from build123d import *

# Parameters (mm, degrees)
F0_R     = 1.75
F1_DEPTH = 1.6
F2_W     = 5.842995
F2_H     = 15.024841
F3_DEPTH = 8
F4_W     = 32
F4_H     = 50
F5_DEPTH = 19
F6_W     = 3
F6_H     = 14
F7_DEPTH = 32
F8_W     = 8.602944
F8_H     = 27.794118
F9_DEPTH = 14


with BuildPart() as f1:
    # F0 (on Top) → F1 (new body)
    with BuildSketch(Plane.XY):
        with BuildLine():
            ThreePointArc((35.5, 25), (34.62132, 27.12132), (32.5, 28))
            Line((32.5, 28), (-32.5, 28))
            ThreePointArc((-32.5, 28), (-34.62132, 27.12132), (-35.5, 25))
            Line((-35.5, 25), (-35.5, -25))
            ThreePointArc((-35.5, -25), (-34.62132, -27.12132), (-32.5, -28))
            Line((-32.5, -28), (32.5, -28))
            ThreePointArc((32.5, -28), (34.62132, -27.12132), (35.5, -25))
            Line((35.5, -25), (35.5, 25))
        make_face()
        with Locations((-32.5, -25)):
            Circle(F0_R, mode=Mode.SUBTRACT)
        with Locations((32.5, -25)):
            Circle(F0_R, mode=Mode.SUBTRACT)
        with Locations((-32.5, 25)):
            Circle(F0_R, mode=Mode.SUBTRACT)
        with Locations((32.5, 25)):
            Circle(F0_R, mode=Mode.SUBTRACT)
    extrude(amount=F1_DEPTH)

    # F2 (on face) → F3 (join)
    with BuildSketch(Plane.XY.offset(1.6)):
        with Locations((25.289628, -6.157123)):
            Rectangle(F2_W, F2_H)
    extrude(amount=F3_DEPTH)

    # F4 (on face) → F5 (join)
    with BuildSketch(Plane.XY.offset(1.6)):
        with Locations((-4.5, 0)):
            Rectangle(F4_W, F4_H)
    extrude(amount=F5_DEPTH)

    # F6 (on face) → F7 (cut, through all)
    with BuildSketch(Plane.YZ.offset(11.5)):
        with Locations((-21.737268, 13.6)):
            Rectangle(F6_W, F6_H)
        with Locations((-16.906764, 13.6)):
            Rectangle(F6_W, F6_H)
        with Locations((-12.07626, 13.6)):
            Rectangle(F6_W, F6_H)
        with Locations((-7.245756, 13.6)):
            Rectangle(F6_W, F6_H)
        with Locations((-2.415252, 13.6)):
            Rectangle(F6_W, F6_H)
        with Locations((2.415252, 13.6)):
            Rectangle(F6_W, F6_H)
        with Locations((7.245756, 13.6)):
            Rectangle(F6_W, F6_H)
        with Locations((12.07626, 13.6)):
            Rectangle(F6_W, F6_H)
        with Locations((16.906764, 13.6)):
            Rectangle(F6_W, F6_H)
        with Locations((21.737268, 13.6)):
            Rectangle(F6_W, F6_H)
    extrude(amount=-F7_DEPTH, mode=Mode.SUBTRACT)

    # F8 (on face) → F9 (join)
    with BuildSketch(Plane.XY.offset(1.6)):
        with Locations((-27.370911, 7.468621)):
            Rectangle(F8_W, F8_H)
    extrude(amount=F9_DEPTH)


solid = f1.part
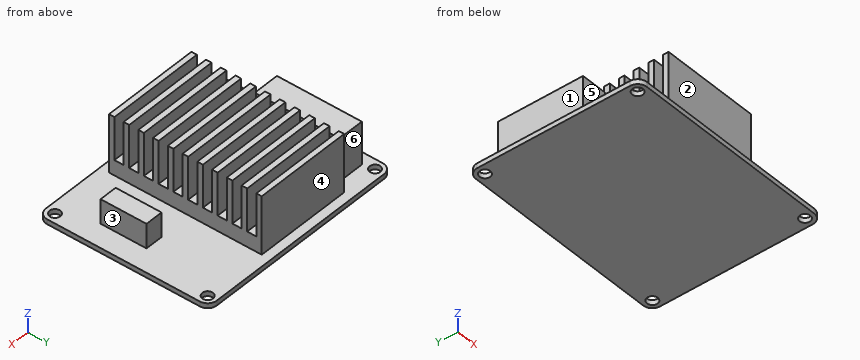
Geometry check sheet. Reference: the model listing, model coordinates, mm. Face numbers are marked on the shaded views. A direction names the side the tool comes from. Coordinates: 2 decimals unless noted, no trailing zeros. Order: outer loops, then holes, each group sorted by start corner. A loop starts at its lowest first (then second) coordinate and runs counter-clockwise, first axis right, second up. Notation, with made-up numbers: (-9.75, 20) - (45.25, 20) arc R33 ccw to (45.25, 54) - close; hole circle Ø1 at (89.5, -40). An arc over 180 degrees is marked (long way). Answer in a Markdown table with one row per item. Add a question column.
1) Cross-section at D-D, the plane y = 8. Record the cut outline in (x, z).
2) Gauge pin test, flat ends, axial feed: P1, Ø1.5, axis at x = -24, z = 13.5, coming from the +Y side; P2, Ø1.5, axis at x = -3.5, y = 7, coming from the +Z side; P3, Ø7, axis at x = 3, z = 14.5, coming from the +Y side. Record the tip position at first contact, or that the pin passes through.
3) Cross-section at B-B, the plane z = 18. State how many separate pieces and enclosed holes the cut face has, then the cut area to 3 significant figures.
4) Cross-section at A-A, the plane x = -26.5. Record the cut outline in (y, z).
5) Set-up check for the marked faces 4, 5 and 6: record each of +Z, -Z, +X, -X, +Y, -Y from which the full face is reachable in a straight line by a thin tool's end or side.
6) Release check for a two-part mould opening along X. For the marked faces 1, 2 and 3 record: +X half, -X half, draft (parallel to the pull), parting line (faces both ways), or undercut.
7) Material ranges on line 1 along Y through (x, z) = (32.5, 0.75); line 2 along X through (y, z) = (8, 3.75); line 3 along Z through (x, y) = (-6.5, 26.5), recorded low to high. Write a range as [from, to].
Check result:
| question | item | result |
|---|---|---|
| 1 | outline | (-35.5, 0) - (35.5, 0) - (35.5, 1.6) - (11.5, 1.6) - (11.5, 6.6) - (-20.5, 6.6) - (-20.5, 1.6) - (-23.07, 1.6) - (-23.07, 15.6) - (-31.67, 15.6) - (-31.67, 1.6) - (-35.5, 1.6) - close |
| 2 | P1 | stops at y = 21.37 |
| 2 | P2 | stops at z = 6.6 |
| 2 | P3 | stops at y = 25 |
| 3 | separate pieces | 11 |
| 3 | enclosed holes | 0 |
| 3 | area | 640 mm² |
| 4 | outline | (-28, 0) - (28, 0) - (28, 1.6) - (21.37, 1.6) - (21.37, 15.6) - (-6.43, 15.6) - (-6.43, 1.6) - (-28, 1.6) - close |
| 5 | face 4 | +Z, +X, -X, +Y |
| 5 | face 5 | +Z, -X, -Y |
| 5 | face 6 | +Z, -X, +Y |
| 6 | face 1 | -X half |
| 6 | face 2 | draft |
| 6 | face 3 | +X half |
| 7 | line 1 | y = [-28, -26.75], [-23.25, 23.25], [26.75, 28] |
| 7 | line 2 | x = [-31.67, -23.07], [-20.5, 11.5] |
| 7 | line 3 | z = [0, 1.6] |
